Check sheet for the modelled part. Datum: model origin and axes. Units: mm. A direction names the side the tool comes from. Give positions to 0.01 mm unless a question says otherwise; leave off trailing zeros. Loops run counter-clockwise (first coordinate to the right, second up) from the corner with the lowest first, then second, coordinate; pieces in that order, holes last. Notation, with made-up numbers: (-2, 29) - (39, 29) arc R20 ccw to (39, 63) - close; hole circle Ø6 at (15.5, -29). An arc over 180 degrees is marked (long way). Use one line per item in the form item = value.
from build123d import *

# Parameters (mm, degrees)
SKETCH1_W           = 65
SKETCH1_H           = 54
BOSS_EXTRUDE1_DEPTH = 25
SKETCH2_W           = 55
SKETCH2_H           = 34
CUT_EXTRUDE1_DEPTH  = 20
SKETCH3_R           = 2
CUT_EXTRUDE2_DEPTH  = 66
FILLET1_R           = 5


with BuildPart() as part:
    # Sketch1 → Boss-Extrude1 (new body)
    with BuildSketch(Plane(origin=(0, 0, 0), x_dir=(1, 0, 0), z_dir=(0, 1, 0))):
        with Locations((32.5, 27)):
            Rectangle(SKETCH1_W, SKETCH1_H)
    extrude(amount=BOSS_EXTRUDE1_DEPTH)

    # Sketch2 → Cut-Extrude1 (cut)
    with BuildSketch(Plane(origin=(0, 25, 0), x_dir=(1, 0, 0), z_dir=(0, 1, 0))):
        with Locations((27.5, 27)):
            Rectangle(SKETCH2_W, SKETCH2_H)
    extrude(amount=-CUT_EXTRUDE1_DEPTH, mode=Mode.SUBTRACT)

    # Sketch3 → Cut-Extrude2 (cut, through all)
    with BuildSketch(Plane(origin=(65, 0, 0), x_dir=(0, 0, -1), z_dir=(1, 0, 0))):
        with Locations((27, 19.64)):
            Circle(SKETCH3_R)
    extrude(amount=-CUT_EXTRUDE2_DEPTH, mode=Mode.SUBTRACT)

    # Fillet1
    fillet1_edges = [part.edges().sort_by_distance(p)[0] for p in [
        (55, 15, -44),
        (55, 15, -10),
    ]]
    fillet(fillet1_edges, radius=FILLET1_R)


solid = part.part
Item 1: Section check D-D on z = -42. Record the boundary of the cut face in (x, y), then the cut area to 3 significant figures.
Answer block:
outline = (0, 0) - (65, 0) - (65, 25) - (54, 25) - (54, 5) - (0, 5) - close
area = 545 mm2
Item 2: Thickness scan on L1, parallel to Z at x = 47.5, y = 17.75; L2, parallel to Y at x = 61.5, z = -27; L3, parallel to X at y = 6, z = -16. Record the ranges inside material, lowest first.
Answer block:
L1 = -54 to -44, -10 to 0
L2 = 0 to 17.64, 21.64 to 25
L3 = 55 to 65
Item 3: Section check A-A on y = 19.64. Record the boundary of the cut face in (x, z).
Answer block:
outline = (0, -54) - (65, -54) - (65, -29) - (55, -29) - (55, -39) arc R5 cw to (50, -44) - (0, -44) - close; (0, -10) - (50, -10) arc R5 cw to (55, -15) - (55, -25) - (65, -25) - (65, 0) - (0, 0) - close
Item 4: Gauge pin test, flat ends, axial feed: P1, Ø10, axis at x = 37, y = 13, coming from the +Z side; P2, Ø1.5, axis at x = 37, z = -28, coming from the +Y side. Record the tip position at first contact, or that the pin passes through.
Answer block:
P1 = 0
P2 = 5
Item 5: Section check B-B on z = -27. Record the boundary of the cut face in (x, y).
Answer block:
outline = (0, 0) - (65, 0) - (65, 17.64) - (55, 17.64) - (55, 5) - (0, 5) - close; (55, 21.64) - (65, 21.64) - (65, 25) - (55, 25) - close
Item 6: Section check C-C on x = 15. Record the boundary of the cut face in (y, z), then the cut area to 3 significant figures.
Answer block:
outline = (0, -54) - (25, -54) - (25, -44) - (5, -44) - (5, -10) - (25, -10) - (25, 0) - (0, 0) - close
area = 670 mm2
Item 7: Access from +Z, -Z, +X, -X, +Y, -Y to the whole of each face (thin tool, end or side, straight path). Record for faces 1 (the face through (53, 15, -43)), 2 (the face through (32, 12, 0)).
Answer block:
face_1 = -X, +Y
face_2 = +Z, +X, -X, +Y, -Y
Item 8: Mould release check, pull along Z, two halves, no side actions. Record for faces 3 (the face through (25, 15, -44)), 4 (the face through (32, 12, -54)), 5 (the face through (65, 12, -27)): released by +Z, released by -Z, zero draft, split by the parting line, or undercut.
Answer block:
face_3 = undercut
face_4 = released by -Z
face_5 = zero draft
